Geometry: final body of the model. Coordinates: model frame, mm. Give positions to 0.01 mm unless a question says otherwise; leave off trailing zeros. Write each loop counter-clockwise with the first axis right and the second up, starting at its lowest first coordinate (ties: lowest second). Pieces come first, ordered by that corner, then holes. Notation, with made-up numbers: (7, 44.5) -> (35, 44.5) arc R20 cw to (35, 71.5) -> close; hole circle Ø5 at (46, 38.25). An arc over 180 degrees is marked (long way). Answer as a JSON object with one key per item and string values. Group by question number.
(1) Section query A-A on z = 38.1. Output: boundary loops of the cut face in (x, y).
(2) Contact query for a flat-ended pin moving along its axis: pin 1 Ø3 at (x, y) = (1, 56) entering from -Z. Output: stop coordinate, or through.
(3) Material intervals for probe 1 along Z at (x, y) = (2, 57.15); probe 2 along Y at (x, z) = (2, 42), sorted ascending.
(4) Section query B-B on y = 57.15. Output: boundary loops of the cut face in (x, z), plus the area to 3 significant figures.
Autodesk Inventor part; units mm, degrees
ref_plane "YZ Plane" through (0, 0, 0) normal (1, 0, 0) x (0, 1, 0)
ref_plane "XZ Plane" through (0, 0, 0) normal (0, 1, 0) x (-1, 0, 0)
ref_plane "XY Plane" through (0, 0, 0) normal (0, 0, 1) x (1, 0, 0)
sketch "Sketch1" plane through (0, 0, 0) normal (1, 0, 0) x (0, 1, 0)
  line L0 (0, 0) -> (69.85, 0)
  line L1 (69.85, 0) -> (69.85, 76.2)
  line L2 (69.85, 76.2) -> (0, 76.2)
  line L3 (0, 76.2) -> (0, 0)
  circle A0 centre (57.15, 38.1) radius 4.7625
  dimension "d0" = 76.2
  dimension "d1" = 69.85
  dimension "d2" = 38.1
  dimension "d3" = 9.525
  dimension "d4" = 12.7
extrude "Extrusion1" add sketch "Sketch1" along normal blind 6.35
properties part number "RollerMountRepresentation"
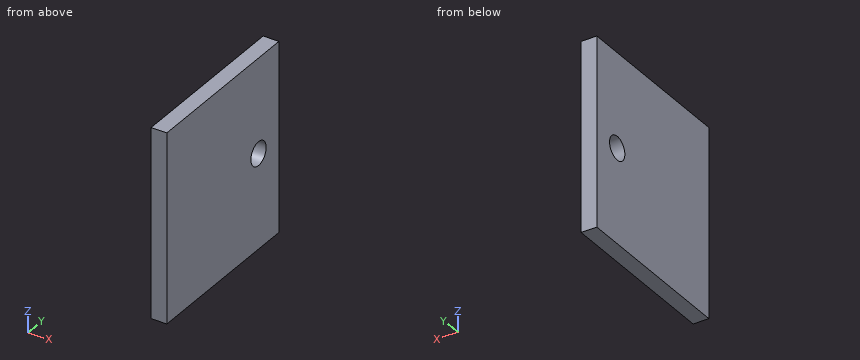
Answer list:
{
 "1": {"outline": "(0, 0) -> (6.35, 0) -> (6.35, 52.39) -> (0, 52.39) -> close; (0, 61.91) -> (6.35, 61.91) -> (6.35, 69.85) -> (0, 69.85) -> close"},
 "2": {"pin 1": "z = 0"},
 "3": {"probe 1": "0 to 33.34, 42.86 to 76.2", "probe 2": "0 to 54.42, 59.88 to 69.85"},
 "4": {"outline": "(0, 0) -> (6.35, 0) -> (6.35, 33.34) -> (0, 33.34) -> close; (0, 42.86) -> (6.35, 42.86) -> (6.35, 76.2) -> (0, 76.2) -> close", "area": "423 mm2"}
}
